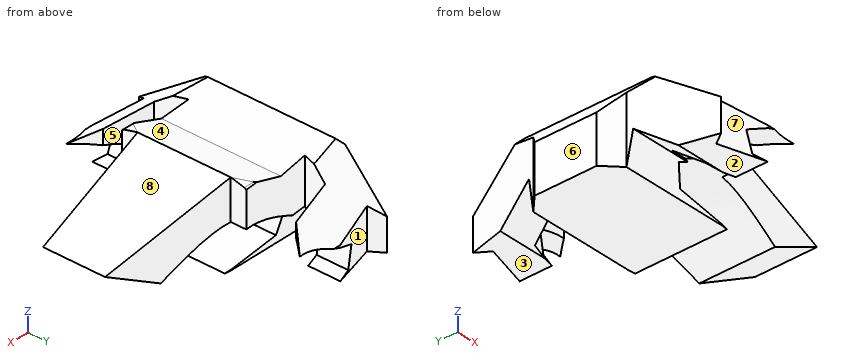
from build123d import *

# Parameters (mm, degrees)
F0_W     = 50
F0_H     = 50
F1_DEPTH = 50
F5_DEPTH = 50
F6_DEPTH = 50
F7_DEPTH = 50


with BuildPart() as f1:
    # F0 (on Top) → F1 (new body)
    with BuildSketch(Plane.XY):
        Rectangle(F0_W, F0_H)
    extrude(amount=F1_DEPTH)

    # F4 (on face) → F5 (cut)
    with BuildSketch(Plane.XY.offset(50)):
        Polygon((-21.7674206942, -9.375), (-25, -6.2522464432), (-25, -25), (-17.8532954305, -25), align=None)
        Polygon((-17.8532954305, -25), (-7.2292452678, -25), (-16.1449728927, -22.4763174233), align=None)
        Polygon((-25, 25), (-25, 6.2522464432), (-21.7674206942, 9.375), (-17.8532954305, 25), align=None)
        Polygon((-7.2292452678, 25), (-17.8532954305, 25), (-16.1449728927, 22.4763174233), align=None)
        Polygon((0, 9.375), (25, 6.25), (25, 25), (1.6374464612, 25), (-3.4748809412, 19.4482598454), (-12.5812105834, 17.2116179019), (-14.1788134351, 11.6998916492), (0, 12.5), align=None)
        Polygon((25, -6.25), (0, -9.375), (0, -12.5), (-14.1788134351, -11.6998916492), (-12.5812105834, -17.2116179019), (-3.4748809412, -19.4482598454), (1.6374464612, -25), (25, -25), align=None)
    extrude(amount=-F5_DEPTH, mode=Mode.SUBTRACT)

    # F2 (on face) → F6 (cut)
    with BuildSketch(Plane(origin=(0, 25, 0), x_dir=(-1, 0, 0), z_dir=(0, 1, 0))):
        Polygon((-25, 50), (-25, 25), (0, 32.1414284285), (8.3757676184, 29.4250827283), (19.8619887233, 30.9700127691), (25, 25), (25, 50), align=None)
        with BuildLine():
            Line((-13.9249656349, 19.0807655454), (-25, 25))
            Line((-25, 25), (-25, 0))
            Line((-25, 0), (25, 0))
            Line((25, 0), (25, 15.3191965073))
            Line((25, 15.3191965073), (-1.6326936893, 15.3191965073))
            Line((-1.6326936893, 15.3191965073), (9.9206976593, 17.0656405389))
            Line((9.9206976593, 17.0656405389), (10.9954318032, 21.0958924145))
            add(Edge.make_bspline(
                [(-13.9249656349, 19.0807655454), (-9.159473278, 21.5130057184), (-0.2120971707, 26.0796204523), (7.4256507336, 22.683291211), (10.9954318032, 21.0958924145)],
                knots=[0, 0, 0, 0, 0.5326133941, 1, 1, 1, 1], degree=3))
        make_face()
    extrude(amount=-F6_DEPTH, mode=Mode.SUBTRACT)

    # F3 (on face) → F7 (cut)
    with BuildSketch(Plane.YZ.offset(25)):
        Polygon((-25, 50), (-25, 23.1785289943), (-12.1138873269, 31.4618550395), (-6.5010248844, 32.8950696164), (0, 32.8950696164), (6.5010248844, 32.8950696164), (12.1138873269, 31.4618550395), (25, 23.1785289943), (25, 50), align=None)
        Polygon((-17.9481003433, 16.6653934866), (-25, 16.6653934866), (-25, 0), (25, 0), (25, 16.6653934866), (17.9481003433, 16.6653934866), (10.4906205088, 21.9307970256), (9.3806944788, 15.3860524297), (0, 15.3860524297), (-9.3806944788, 15.3860524297), (-10.4906205088, 21.9307970256), align=None)
    extrude(amount=-F7_DEPTH, mode=Mode.SUBTRACT)


solid = f1.part
The model under review builds one solid part; all positions refer to its coordinate system, in mm. Face numbers are marked on the shaded views. A direction names the side the tool comes from. Give positions to 0.01 mm unless a question says otherwise; leave off trailing zeros. Order: outer loops, then holes, each group sorted by start corner. A loop starts at its lowest first (then second) coordinate and runs counter-clockwise, first axis right, second up. Notation, with made-up numbers: M 41.5,29.5 L 79.5,29.5 A27 cw 79.5,57.5 Z; hole C 31.5,66 d2. An arc over 180 degrees is marked long. One line per question, with ' | ' between items. Start each with the question number.
1) Consider section A-A, the plane z = 18. Give the boundary of the cut face in (x, y) (3 decimals).
2) For the marked faces 1, 2, 3, 4 and 5, list the 3-axis set-ups (+Z, -Z, +X, -X, +Y, -Y) from which the entire face can be reached by the end or side of a thin tool; tool diameter is ignored.
3) Consider section C-C, the plane z = 26. Give the boundary of the cut face in (x, y) (3 decimals), then the cut area to 3 significant figures.
4) Wall thickness on L1, parallel to Y at x = -9.5, z = 23.75; L2, parallel to Y at x = -12.5, z = 20.5; L3, parallel to X at y = 1.5, z = 19.75: over which ranges is each line inside the solid? List them lowest first. Write a range as from..to.
5) Consider section D-D, the plane x = 19.5. Give the boundary of the cut face in (y, z).
6) Clearance check with flat-ended pins moving along their axes: P1, Ø12, axis at x = 13, y = -18, coming from the -Z side; P2, Ø5, axis at x = 7.5, z = 19.5, coming from the -Y side; P3, Ø4, axis at y = 11.5, z = 19.5, coming from the -X side; P4, Ø3.5, axis at x = -13.5, y = -21.5, coming from the -Z side. State where each tip first meets the part, or that it passes through.
7) Consider section B-B, the plane x = -4.5. State how many separate pieces and enclosed holes the cut face has, then the cut area to 3 significant figures.
8) Mouldability with a two-part tool opening along X and no side actions: class the marked faces 6, 7 and 8 as pulls with the +X half, pulls with the -X half, needs draft (parallel to the pull), parting line crosses it, or undercut.
Found:
1) outline: M -25,-6.252 L -21.767,-9.375 L -21.655,-9.824 L -10.17,-9.824 L -10.17,9.824 L -21.655,9.824 L -21.767,9.375 L -25,6.252 Z; M -20.093,-16.058 L -17.853,-25 L -16.145,-22.476 L -10.17,-24.168 L -10.17,-17.804 L -12.581,-17.212 L -12.916,-16.058 Z; M -20.093,16.058 L -12.916,16.058 L -12.581,17.212 L -10.17,17.804 L -10.17,24.168 L -16.145,22.476 L -17.853,25 Z
2) face 1: +Z, -Z, +Y | face 2: -Z, +X, -X, -Y | face 3: -Z, +X, -X, +Y | face 4: +Z, +Y, -Y | face 5: +Z, -Z, +X
3) outline: M -24.139,-7.084 L -21.767,-9.375 L -18.953,-20.611 L -2.404,-20.611 L -3.475,-19.448 L -12.581,-17.212 L -14.179,-11.7 L 0,-12.5 L 0,-9.375 L 21.499,-6.688 L 21.499,6.688 L 0,9.375 L 0,12.5 L -14.179,11.7 L -12.581,17.212 L -3.475,19.448 L -2.404,20.611 L -18.953,20.611 L -21.767,9.375 L -24.139,7.084 Z | area: 1,070 mm²
4) L1: y = -24.11..-17.97, -11.96..11.96, 17.97..24.11 | L2: y = -23.51..-17.23, -10.25..10.25, 17.23..23.51 | L3: x = -25..-10.64, 12.61..15.18
5) outline: M -6.94,22.06 L 6.94,22.06 L 6.94,26.57 L -6.94,26.57 Z
6) P1: passes through | P2: stops at y = -8.37 | P3: stops at x = -21.74 | P4: stops at z = 16.67
7) separate pieces: 4 | enclosed holes: 0 | area: 207 mm²
8) face 6: pulls with the -X half | face 7: undercut | face 8: pulls with the +X half
